```python
from build123d import *

# Parameters (mm, degrees)
F0_R     = 25.4
F0_R_2   = 6.35
F1_DEPTH = 1.524
F2_W     = 2.667
F2_H     = 8.255
F3_DEPTH = 73
F4_R     = 0.8128


# Not quite as in the source:
# - an extrude ends at something that could not be found from the text; its depth is read off the source's solid


with BuildPart() as f1:
    # F0 (on Front) → F1 (new body)
    with BuildSketch(Plane.XZ):
        Circle(F0_R)
        Circle(F0_R_2, mode=Mode.SUBTRACT)
    extrude(amount=F1_DEPTH)

    # F2 (on Front) → F3 (cut, through all)
    with BuildSketch(Plane.XZ):
        with Locations((0, 4.1275)):
            Rectangle(F2_W, F2_H)
    extrude(amount=F3_DEPTH, mode=Mode.SUBTRACT)

    # F4
    f4_edges = [f1.edges().sort_by_distance(p)[0] for p in [
        (-1.3335, -0.762, 8.255),
        (1.3335, -0.762, 8.255),
    ]]
    fillet(f4_edges, radius=F4_R)


solid = f1.part
```
Geometry check sheet. Reference: the model listing, model coordinates, mm. A direction names the side the tool comes from. Coordinates: 2 decimals unless noted, no trailing zeros. Write each loop counter-clockwise with the first axis right and the second up, starting at its lowest first coordinate (ties: lowest second). Pieces come first, ordered by that corner, then holes. Notation, with made-up numbers: M 21.5,63 L 63.5,63 A28 cw 63.5,97 Z; hole C 60.25,-19.5 d6. An arc over 180 degrees is marked long. Answer as a JSON object with one key per item and string values.
1. Section check D-D, the plane x = 19.5. Enter the section's corners in (y, z).
Answers below:
{"outline": "M -1.52,-16.28 L 0,-16.28 L 0,16.28 L -1.52,16.28 Z"}
2. Draft check along Z on faces 3 (the flat face through (5, -1.524, -5)), 4 (the cylindrical face through (-5.506, -0.751, -24.796)), 5 (the flat face through (-1.334, -1, 7)). Enter one of: released by +Z, released by -Z, zero draft, split by the parting line, or undercut.
Answers below:
{"face 3": "zero draft", "face 4": "split by the parting line", "face 5": "undercut"}
3. Scan lines: L1, parallel to Z at x = 0, y = -0.9 (3 decimals); L2, parallel to Z at x = 1, y = -0.55; L3, parallel to Z at x = -20, y = -1.3. Record each from-to range of solid material in increasing order.
Answers below:
{"L1": "z = -25.4 to -6.35, 8.255 to 25.4", "L2": "z = -25.38 to -6.27, 8.1 to 25.38", "L3": "z = -15.66 to 15.66"}
4. Tool access check on faces 1 (the flat face through (5, 0, -5)), 2 (the flat face through (1.334, -1, 7)). Record the directions out of +Z, -Z, +X, -X, +Y, -Y that give a thin tool (end or side, any length) a straight path to the whole face; none if there is none.
Answers below:
{"face 1": "+Z, -Z, +X, -X, +Y", "face 2": "+Y, -Y"}
5. Section check A-A, the plane z = 0. Enter the section's corners in (x, y).
Answers below:
{"outline": "M -25.4,-1.52 L -6.35,-1.52 L -6.35,0 L -25.4,0 Z; M 6.35,-1.52 L 25.4,-1.52 L 25.4,0 L 6.35,0 Z"}
6. Section check C-C, the plane z = -20. Enter the section's corners in (x, y).
Answers below:
{"outline": "M -15.66,-1.52 L 15.66,-1.52 L 15.66,0 L -15.66,0 Z"}
